```python
from build123d import *

# Parameters (mm, degrees)
BOSS_EXTRUDE3_DEPTH = 8
FILLET1_R           = 8
CUT_EXTRUDE3_DEPTH  = 10


with BuildPart() as part:
    # Sketch2 → Boss-Extrude3 (new body)
    with BuildSketch(Plane.XY.offset(-1552.384718604)):
        Polygon((-493.118842126, 700), (-493.118842126, 560), (-480.118842126, 560), (38.881157874, 560), (38.881157874, 700), (-480.118842126, 700), align=None)
        with BuildLine():
            Line((15.631157874, 584.25), (15.631157874, 675.75))
            ThreePointArc((15.631157874, 675.75), (19.881157874, 680), (24.131157874, 675.75))
            Line((24.131157874, 675.75), (24.131157874, 584.25))
            ThreePointArc((24.131157874, 584.25), (19.881157874, 580), (15.631157874, 584.25))
        make_face(mode=Mode.SUBTRACT)
        with BuildLine():
            Line((-15.868842127, 584.25), (-15.868842127, 675.75))
            ThreePointArc((-15.868842127, 675.75), (-20.118842127, 680), (-24.368842127, 675.75))
            Line((-24.368842127, 675.75), (-24.368842127, 584.25))
            ThreePointArc((-24.368842127, 584.25), (-20.118842127, 580), (-15.868842127, 584.25))
        make_face(mode=Mode.SUBTRACT)
        with BuildLine():
            Line((-438.368842126, 584.25), (-438.368842126, 675.75))
            ThreePointArc((-438.368842126, 675.75), (-434.118842126, 680), (-429.868842126, 675.75))
            Line((-429.868842126, 675.75), (-429.868842126, 584.25))
            ThreePointArc((-429.868842126, 584.25), (-434.118842126, 580), (-438.368842126, 584.25))
        make_face(mode=Mode.SUBTRACT)
        with BuildLine():
            Line((-469.868842126, 584.25), (-469.868842126, 675.75))
            ThreePointArc((-469.868842126, 675.75), (-474.118842126, 680), (-478.368842126, 675.75))
            Line((-478.368842126, 675.75), (-478.368842126, 584.25))
            ThreePointArc((-478.368842126, 584.25), (-474.118842126, 580), (-469.868842126, 584.25))
        make_face(mode=Mode.SUBTRACT)
    extrude(amount=BOSS_EXTRUDE3_DEPTH)

    # Fillet1
    fillet1_edges = [part.edges().sort_by_distance(p)[0] for p in [
        (-493.118842126, 560, -1548.384718604),
        (-493.118842126, 700, -1548.384718604),
        (38.881157874, 700, -1548.384718604),
        (38.881157874, 560, -1548.384718604),
    ]]
    fillet(fillet1_edges, radius=FILLET1_R)

    # Sketch7 → Cut-Extrude3 (cut)
    with BuildSketch(Plane.XY.offset(-1544.384718604)):
        with BuildLine():
            Line((-256.068842126, 675.75), (-256.068842126, 584.25))
            ThreePointArc((-256.068842126, 584.25), (-260.243842126, 580.075), (-264.418842126, 584.25))
            Line((-264.418842126, 584.25), (-264.418842126, 675.75))
            ThreePointArc((-264.418842126, 675.75), (-260.243842126, 679.925), (-256.068842126, 675.75))
        make_face()
        with BuildLine():
            Line((-197.668842126, 675.75), (-197.668842126, 584.25))
            ThreePointArc((-197.668842126, 584.25), (-193.493842126, 580.075), (-189.318842126, 584.25))
            Line((-189.318842126, 584.25), (-189.318842126, 675.75))
            ThreePointArc((-189.318842126, 675.75), (-193.493842126, 679.925), (-197.668842126, 675.75))
        make_face()
    extrude(amount=-CUT_EXTRUDE3_DEPTH, mode=Mode.SUBTRACT)


solid = part.part
```
Geometry check sheet. Reference: the model listing, model coordinates, mm. Round coordinates to 2 decimals unless told otherwise and drop trailing zeros. Order: outer loops, then holes, each group sorted by start corner. A loop starts at its lowest first (then second) coordinate and runs counter-clockwise, first axis right, second up. Notation, with made-up numbers: M -7.75,67 L 47.25,67 A21 cw 47.25,89 Z; hole C -26.5,81.25 d6. An arc over 180 degrees is marked long. Answer as CSV lines item,"result".
1) Sectioned sample at B-B on z = -1548. Give the number of separate pieces and of enclosed holes in the cut face, and give its area (3 significant figures).
Entries:
separate pieces,"1"
enclosed holes,"6"
area,"69,400 mm2"
2) Sectioned sample at A-A on y = 649. Record the cut outline in (x, z).
Entries:
outline,"M -493.12,-1552.38 L -478.37,-1552.38 L -478.37,-1544.38 L -493.12,-1544.38 Z; M -469.87,-1552.38 L -438.37,-1552.38 L -438.37,-1544.38 L -469.87,-1544.38 Z; M -429.87,-1552.38 L -264.42,-1552.38 L -264.42,-1544.38 L -429.87,-1544.38 Z; M -256.07,-1552.38 L -197.67,-1552.38 L -197.67,-1544.38 L -256.07,-1544.38 Z; M -189.32,-1552.38 L -24.37,-1552.38 L -24.37,-1544.38 L -189.32,-1544.38 Z; M -15.87,-1552.38 L 15.63,-1552.38 L 15.63,-1544.38 L -15.87,-1544.38 Z; M 24.13,-1552.38 L 38.88,-1552.38 L 38.88,-1544.38 L 24.13,-1544.38 Z"
3) Thickness scan on probe 1 along Y at (x, z) = (-260, -1550.25). Record the ranges inside material, lowest first. Write a range as [from, to].
Entries:
probe 1,"[560, 580.08], [679.92, 700]"
